CAD build for the part. Positions are in the model's coordinates, mm. A direction names the side the tool comes from. Round coordinates to 2 decimals unless told otherwise and drop trailing zeros. Write each loop counter-clockwise with the first axis right and the second up, starting at its lowest first coordinate (ties: lowest second). Pieces come first, ordered by that corner, then holes. Notation, with made-up numbers: (16, -22) - (55, -22) arc R29 ccw to (55, 13) - close; hole circle Ø10 at (60, 43). An arc over 180 degrees is marked (long way). Answer in a Markdown table with one row per item.
```python
from build123d import *

# Parameters (mm, degrees)
SKETCH1_W                = 60
SKETCH1_H                = 27
BOSS_EXTRUDE1_DEPTH      = 6
CUT_EXTRUDE19_DEPTH      = 67.068146637
CUT_EXTRUDE19_DEPTH_BACK = 67.068146637
SKETCH9_W                = 2.8
SKETCH9_H                = 11.5
CUT_EXTRUDE20_DEPTH      = 67.068146637
CUT_EXTRUDE21_DEPTH      = 67.068146637
CUT_EXTRUDE21_DEPTH_BACK = 67.068146637
SKETCH10_W               = 2.8
SKETCH10_H               = 9.5
M5_TAPPED_HOLE3_D        = 4.2
M5_TAPPED_HOLE3_DEPTH    = 12.4
M5_TAPPED_HOLE3_TIP      = 1.2618073
M5_TAPPED_HOLE4_D        = 4.2
M5_TAPPED_HOLE4_DEPTH    = 12.4
M5_TAPPED_HOLE4_TIP      = 1.2618073


with BuildPart() as part:
    # Sketch1 → Boss-Extrude1 (new body)
    with BuildSketch(Plane(origin=(0, 0, 0), x_dir=(0, 0, -1), z_dir=(1, 0, 0))):
        with Locations((30, 13.5)):
            Rectangle(SKETCH1_W, SKETCH1_H)
    extrude(amount=BOSS_EXTRUDE1_DEPTH)

    # 3DSketch1 → Cut-Extrude19 (cut, two sides: drawn at the far end of the back side and taken through both)
    with BuildSketch(Plane(origin=(6, 27, 0), x_dir=(-0.24253562503633286, -0.970142500145332, 0), z_dir=(0, 0, -1)).offset(-CUT_EXTRUDE19_DEPTH_BACK)):
        Polygon((0, 0), (0.363803438, 1.45521375), (6.184658438, 0), (5.820855001, -1.45521375), align=None)
    extrude(amount=CUT_EXTRUDE19_DEPTH + CUT_EXTRUDE19_DEPTH_BACK, mode=Mode.SUBTRACT)

    # Sketch9 → Cut-Extrude20 (cut, through all)
    with BuildSketch(Plane(origin=(0, 0, -60), x_dir=(-1, 0, 0), z_dir=(0, 0, -1))):
        with Locations((-1.4, 5.75)):
            Rectangle(SKETCH9_W, SKETCH9_H)
    extrude(amount=-CUT_EXTRUDE20_DEPTH, mode=Mode.SUBTRACT)

    # Sketch10 → Cut-Extrude21 (cut, two sides: drawn at the far end of the back side and taken through both)
    with BuildSketch(Plane(origin=(0, 0, -60), x_dir=(-1, 0, 0), z_dir=(0, 0, -1)).offset(-CUT_EXTRUDE21_DEPTH_BACK)):
        with Locations((-1.4, 22.25)):
            Rectangle(SKETCH10_W, SKETCH10_H)
    extrude(amount=CUT_EXTRUDE21_DEPTH + CUT_EXTRUDE21_DEPTH_BACK, mode=Mode.SUBTRACT)

    # M5 Tapped Hole3
    with Locations(Plane(origin=(0, 14.5, -50), x_dir=(0, 0, -1), z_dir=(-1, 0, 0))):
        with Locations((0, 0)):
            Hole(M5_TAPPED_HOLE3_D / 2, depth=M5_TAPPED_HOLE3_DEPTH)
            with Locations((0, 0, -(M5_TAPPED_HOLE3_DEPTH + M5_TAPPED_HOLE3_TIP / 2))):  # 118° drill point
                Cone(0, M5_TAPPED_HOLE3_D / 2, M5_TAPPED_HOLE3_TIP, mode=Mode.SUBTRACT)

    # M5 Tapped Hole4
    with Locations(Plane(origin=(0, 14.5, -10), x_dir=(0, 0, -1), z_dir=(-1, 0, 0))):
        with Locations((0, 0)):
            Hole(M5_TAPPED_HOLE4_D / 2, depth=M5_TAPPED_HOLE4_DEPTH)
            with Locations((0, 0, -(M5_TAPPED_HOLE4_DEPTH + M5_TAPPED_HOLE4_TIP / 2))):  # 118° drill point
                Cone(0, M5_TAPPED_HOLE4_D / 2, M5_TAPPED_HOLE4_TIP, mode=Mode.SUBTRACT)


solid = part.part
```
Q1. Pull direction Y, two halves, no side cores. Call faces 4 (the flat face through (4, 27, -30)), 5 (the cylindrical face through (3.04, 14.41, -12.1)), 6 (the flat face through (4, 13, 0)): released by +Y, released by -Y, zero draft, split by the parting line, or undercut.
Computed:
| item | result |
|---|---|
| face 4 | released by +Y |
| face 5 | undercut |
| face 6 | zero draft |
Q2. Saw through at A-A on z = -50. List the corners of the cut face in (x, y), then the cut area to 3 significant figures.
Computed:
| item | result |
|---|---|
| outline | (0, 11.5) - (2.8, 11.5) - (2.8, 0) - (6, 0) - (6, 12.4) - (0, 12.4) - close; (0, 16.6) - (6, 16.6) - (6, 21) - (4.5, 21) - (4.5, 27) - (2.8, 27) - (2.8, 17.5) - (0, 17.5) - close |
| area | 69.0 mm2 |
Q3. Drill centre lines: line 1 (Z direction, x = 3.1, y = 14.5); line 2 (Y direction, x = 2.85, z = -10); line 3 (Y direction, x = 2.05, z = -50). Where is each one in solid material? Low to high.
Computed:
| item | result |
|---|---|
| line 1 | z = -60 to -52.1, -47.9 to -12.1, -7.9 to 0 |
| line 2 | y = 0 to 12.4, 16.6 to 27 |
| line 3 | y = 11.5 to 12.4, 16.6 to 17.5 |
Q4. Saw through at B-B on y = 14.5. List the corners of the cut face in (x, z).
Computed:
| item | result |
|---|---|
| outline | (0, -60) - (6, -60) - (6, -52.1) - (0, -52.1) - close; (0, -47.9) - (6, -47.9) - (6, -12.1) - (0, -12.1) - close; (0, -7.9) - (6, -7.9) - (6, 0) - (0, 0) - close |
Q5. Flat gauge pins, fed straight in: pin 1 (0.8 mm diameter, centred on x = 1, z = -41, fed in from -Y); pin 2 (6 mm diameter, centred on y = 3.5, z = -17.5, fed in from -X). Where does each tip first touch, or does it go through?
Computed:
| item | result |
|---|---|
| pin 1 | stops at y = 11.5 |
| pin 2 | stops at x = 2.8 |
Q6. Saw through at C-C on x = 3.75. List the corners of the cut face in (y, z).
Computed:
| item | result |
|---|---|
| outline | (0, -60) - (27, -60) - (27, 0) - (0, 0) - close; hole circle Ø4.2 at (14.5, -50); hole circle Ø4.2 at (14.5, -10) |
Q7. 3-axis set-ups, long thin cutter, end or side, ignore diameter. For faces 1 (the flat face through (4.5, 24, -30)), 2 (the flat face through (1, 17.5, -30)), 3 (the flat face through (1, 11.5, -30)): which of +Z, -Z, +X, -X, +Y, -Y reach the whole face in a straight line?
Computed:
| item | result |
|---|---|
| face 1 | +Z, -Z, +X, +Y |
| face 2 | +Z, -Z, -X, +Y |
| face 3 | +Z, -Z, -X, -Y |
Q8. Saw through at D-D on z = -19. List the corners of the cut face in (x, y).
Computed:
| item | result |
|---|---|
| outline | (0, 11.5) - (2.8, 11.5) - (2.8, 0) - (6, 0) - (6, 21) - (4.5, 21) - (4.5, 27) - (2.8, 27) - (2.8, 17.5) - (0, 17.5) - close |
